```python
from build123d import *

# Parameters (mm, degrees)
SKETCH1_R                = 7.5
SKETCH1_R_2              = 2.45
BOSS_EXTRUDE1_DEPTH      = 10
CUT_EXTRUDE1_DEPTH       = 10
FILLET1_R                = 0.5
CIRPATTERN1_COUNT        = 15
FILLET1_OF_CIRPATTERN1_R = 0.5
SKETCH3_R                = 4.45
SKETCH3_R_2              = 2.45
BOSS_EXTRUDE2_DEPTH      = 10


with BuildPart() as part:
    # Sketch1 → Boss-Extrude1 (new body)
    with BuildSketch(Plane.XY):
        Circle(SKETCH1_R)
        Circle(SKETCH1_R_2, mode=Mode.SUBTRACT)
    extrude(amount=BOSS_EXTRUDE1_DEPTH)

    # Sketch2 → Cut-Extrude1 (cut)
    with BuildSketch(Plane(origin=(0, 0, 0), x_dir=(-1, 0, 0), z_dir=(0, 0, -1))):
        Polygon((-0.65, 6), (0.65, 6), (1, 7.5), (-1, 7.5), align=None)
    cut_extrude1 = extrude(amount=-CUT_EXTRUDE1_DEPTH, mode=Mode.SUBTRACT)

    # Fillet1
    fillet1_edges = [part.edges().sort_by_distance(p)[0] for p in [
        (-0.984846702, 7.435057295, 5),
        (0.984846702, 7.435057295, 5),
        (0.65, 6, 5),
        (-0.65, 6, 5),
    ]]
    fillet(fillet1_edges, radius=FILLET1_R)

    # CirPattern1: Cut-Extrude1 ×15 about axis
    cirpattern1_axis = Axis((0, 0, 0), (0, 0, 1))
    for i in range(1, CIRPATTERN1_COUNT):
        add(cut_extrude1.rotate(cirpattern1_axis, i * 360 / CIRPATTERN1_COUNT), mode=Mode.SUBTRACT)

    # Fillet1 of CirPattern1
    fillet1_of_cirpattern1_edges = [part.edges().sort_by_distance(p)[0] for p in [
        (-3.923812476, 6.391689577, 5),
        (-2.124408014, 7.19283606, 5),
        (-1.846615311, 5.745651564, 5),
        (-3.034224406, 5.216893928, 5),
        (-6.184315427, 4.243140665, 5),
        (-4.866333285, 5.706908126, 5),
        (-4.023934059, 4.497827775, 5),
        (-4.893803847, 3.531739502, 5),
        (-7.375494057, 1.360914185, 5),
        (-6.766825321, 3.234203932, 5),
        (-5.505478051, 2.472288702, 5),
        (-5.907200144, 1.235915231, 5),
        (-7.29138276, -1.756626722, 5),
        (-7.497271785, 0.202276495, 5),
        (-6.035074873, 0.019268452, 5),
        (-5.899187871, -1.273610012, 5),
        (-5.946525145, -4.57043091, 5),
        (-6.931371847, -2.864626384, 5),
        (-5.521152423, -2.437083488, 5),
        (-4.871152423, -3.562916512, 5),
        (-3.573459309, -6.593966073, 5),
        (-5.166974747, -5.436209338, 5),
        (-4.05257256, -4.472041552, 5),
        (-3.000850467, -5.23616238, 5),
        (-0.582509895, -7.477344597, 5),
        (-2.509160772, -7.067822311, 5),
        (-1.883266085, -5.733743005, 5),
        (-0.611674204, -6.004028203, 5),
        (2.509160772, -7.067822311, 5),
        (0.582509895, -7.477344597, 5),
        (0.611674204, -6.004028203, 5),
        (1.883266085, -5.733743005, 5),
        (5.166974747, -5.436209338, 5),
        (3.573459309, -6.593966073, 5),
        (3.000850467, -5.23616238, 5),
        (4.05257256, -4.472041552, 5),
        (6.931371847, -2.864626384, 5),
        (5.946525145, -4.57043091, 5),
        (4.871152423, -3.562916512, 5),
        (5.521152423, -2.437083488, 5),
        (7.497271785, 0.202276495, 5),
        (7.29138276, -1.756626722, 5),
        (5.899187871, -1.273610012, 5),
        (6.035074873, 0.019268452, 5),
        (6.766825321, 3.234203932, 5),
        (7.375494057, 1.360914185, 5),
        (5.907200144, 1.235915231, 5),
        (5.505478051, 2.472288702, 5),
        (4.866333285, 5.706908126, 5),
        (6.184315427, 4.243140665, 5),
        (4.893803847, 3.531739502, 5),
        (4.023934059, 4.497827775, 5),
        (2.124408014, 7.19283606, 5),
        (3.923812476, 6.391689577, 5),
        (3.034224406, 5.216893928, 5),
        (1.846615311, 5.745651564, 5),
    ]]
    fillet(fillet1_of_cirpattern1_edges, radius=FILLET1_OF_CIRPATTERN1_R)

    # Sketch3 → Boss-Extrude2 (add)
    with BuildSketch(Plane(origin=(0, 0, 0), x_dir=(-1, 0, 0), z_dir=(0, 0, -1))):
        Circle(SKETCH3_R)
        Circle(SKETCH3_R_2, mode=Mode.SUBTRACT)
    extrude(amount=BOSS_EXTRUDE2_DEPTH)


solid = part.part
```
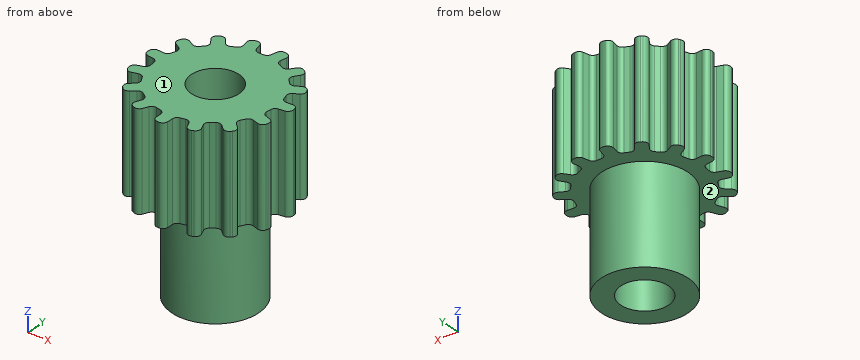
Can you work these out from the model? Positions are in its coordinate system, mm. Face numbers are marked on the shaded views. A direction names the side the tool comes from. Round coordinates to 2 decimals unless told otherwise and drop trailing zeros. Loops run counter-clockwise (first coordinate to the right, second up) from the corner with the lowest first, then second, coordinate; pieces in that order, holes last. Notation, with made-up numbers: M 23,55.5 L 37,55.5 A33 cw 37,86.5 Z; hole C -20.75,-34 d5. An arc over 180 degrees is marked long. Write item = value, one per line. Start each with the question number.
(1) Which directions (+Z, -Z, +X, -X, +Y, -Y) give clear straight access to the entire face, cutting with the end or side of a thin tool? Please do the marked faces 1 and 2.
(2) Suppose I cut it at A-A on z = -1.25. Write out the boundary of the cut face in (x, y), plus the area to 3 significant figures.
(3) I need wall thicknesses on line 1 along Y through (x, z) = (0, -7.75); line 2 along X through (y, z) = (3.75, 8.25); line 3 along Y through (x, z) = (0, 5). Which ranges of each line are inside material? Lowest first, please.
(4) I'm going to push flat-ended pins straight in: P1, Ø3, axis at x = -5.5, z = 2.5, coming from the -Y side; P2, Ø3, axis at y = 0, z = -0.5, coming from the +X side; P3, Ø2, axis at y = 1, z = -1.5, coming from the +X side; P4, Ø1.5, axis at y = -3, z = 3, coming from the +X side. Where does each tip first touch, or does it pass through?
Answer block:
q1.face_1 = +Z, +X, -X, +Y, -Y
q1.face_2 = -Z
q2.outline = C 0,0 d8.9; hole C 0,0 d4.9
q2.area = 43.4 mm²
q3.line_1 = -4.45 to -2.45, 2.45 to 4.45
q3.line_2 = -6.5 to -5.29, -4.72 to 4.72, 5.29 to 6.5
q3.line_3 = -7.5 to -2.45, 2.45 to 6
q4.P1 = -5.25
q4.P2 = 7.47
q4.P3 = 4.45
q4.P4 = 7.15
